Design review of the part built by this model. Coordinates are the model's own, in mm. Give positions to 0.01 mm unless a question says otherwise; leave off trailing zeros. Order: outer loops, then holes, each group sorted by start corner. A loop starts at its lowest first (then second) coordinate and runs counter-clockwise, first axis right, second up. Notation, with made-up numbers: (3.25, 49) -> (10.25, 49) arc R19 cw to (10.25, 61) -> close; hole circle Ø11 at (11, 67). An arc over 180 degrees is marked (long way). One line per item, written item: value. Start each with the question number.
1) Consider section A-A (y = 46.5). State the section outline as (x, z) points.
2) For pin 1 (1.8 mm diameter, centred on x = 0, y = 7.5, fed in from +Z), flat-tipped, find the tip position at first contact; note if it passes through.
3) Wall thickness on line 1 along X through (y, z) = (58, -3.5); line 2 along Y through (x, z) = (0, 6.8): over which ranges is each line inside the solid? List them lowest first. Write a range as from..to.
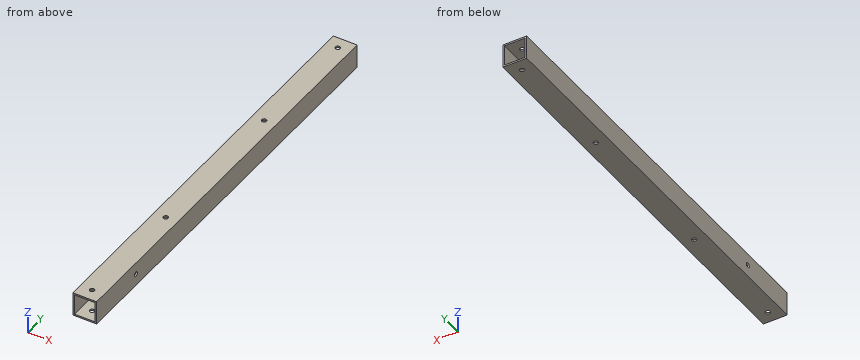
from build123d import *

# Parameters (mm, degrees)
SKETCH_1_W          = 15
SKETCH_1_H          = 15
SKETCH_1_W_2        = 13
SKETCH_1_H_2        = 13
EXTRUDE_1_DEPTH     = 265
SKETCH_2_R          = 1.5
CUT_EXTRUDE_1_DEPTH = 266.530130117
SKETCH_3_R          = 1.5
CUT_EXTRUDE_2_DEPTH = 266.530130117


with BuildPart() as part:
    # 草图1 → 凸台-拉伸1 (new body)
    with BuildSketch(Plane(origin=(0, 0, 0), x_dir=(1, 0, 0), z_dir=(0, 1, 0))):
        Rectangle(SKETCH_1_W, SKETCH_1_H)
        Rectangle(SKETCH_1_W_2, SKETCH_1_H_2, mode=Mode.SUBTRACT)
    extrude(amount=EXTRUDE_1_DEPTH)

    # 草图2 → 切除-拉伸1 (cut, through all)
    with BuildSketch(Plane.XY.offset(7.5)):
        with Locations((0, 7.5)):
            Circle(SKETCH_2_R)
        with Locations((0, 257.5)):
            Circle(SKETCH_2_R)
        with Locations((0, 182.5)):
            Circle(SKETCH_2_R)
        with Locations((0, 82.5)):
            Circle(SKETCH_2_R)
    extrude(amount=-CUT_EXTRUDE_1_DEPTH, mode=Mode.SUBTRACT)

    # 草图3 → 切除-拉伸2 (cut, through all)
    with BuildSketch(Plane(origin=(7.5, 0, 0), x_dir=(0, 0, -1), z_dir=(1, 0, 0))):
        with Locations((0, 40)):
            Circle(SKETCH_3_R)
    extrude(amount=-CUT_EXTRUDE_2_DEPTH, mode=Mode.SUBTRACT)


solid = part.part
Checked values:
1. outline: (-7.5, -7.5) -> (7.5, -7.5) -> (7.5, 7.5) -> (-7.5, 7.5) -> close; hole (-6.5, -6.5) -> (6.5, -6.5) -> (6.5, 6.5) -> (-6.5, 6.5) -> close
2. pin 1: passes through
3. line 1: x = -7.5..-6.5, 6.5..7.5
3. line 2: y = 0..6, 9..81, 84..181, 184..256, 259..265
